```python
from build123d import *

# Parameters (mm, degrees)
SKETCH1_R           = 37.5
SKETCH1_R_2         = 21.5
BOSS_EXTRUDE1_DEPTH = 4
SKETCH2_R           = 29.5
SKETCH2_R_2         = 21.5
BOSS_EXTRUDE2_DEPTH = 79.3
SKETCH3_R           = 1.55
CUT_EXTRUDE1_DEPTH  = 96.399109011
CIRPATTERN1_COUNT   = 3
SKETCH4_R           = 2
CUT_EXTRUDE2_DEPTH  = 6
CIRPATTERN2_COUNT   = 4


with BuildPart() as part:
    # Sketch1 → Boss-Extrude1 (new body)
    with BuildSketch(Plane(origin=(0, 0, 0), x_dir=(1, 0, 0), z_dir=(0, 1, 0))):
        with Locations(Location((0, 0, 0), (0, 0, 270))):
            Circle(SKETCH1_R)
        with Locations(Location((0, 0, 0), (0, 0, 270))):
            Circle(SKETCH1_R_2, mode=Mode.SUBTRACT)
    extrude(amount=BOSS_EXTRUDE1_DEPTH)

    # Sketch2 → Boss-Extrude2 (add)
    with BuildSketch(Plane(origin=(0, 4, 0), x_dir=(1, 0, 0), z_dir=(0, 1, 0))):
        with Locations(Location((0, 0, 0), (0, 0, 270))):
            Circle(SKETCH2_R)
        with Locations(Location((0, 0, 0), (0, 0, 270))):
            Circle(SKETCH2_R_2, mode=Mode.SUBTRACT)
    extrude(amount=BOSS_EXTRUDE2_DEPTH)

    # Sketch3 → Cut-Extrude1 (cut, through all)
    with BuildSketch(Plane(origin=(0, 4, 0), x_dir=(1, 0, 0), z_dir=(0, 1, 0))):
        with Locations(Location((0, 33.5, 0), (0, 0, 270))):
            Circle(SKETCH3_R)
    cut_extrude1 = extrude(amount=-CUT_EXTRUDE1_DEPTH, mode=Mode.SUBTRACT)

    # CirPattern1: Cut-Extrude1 ×3 about axis
    cirpattern1_axis = Axis((0, 0, 0), (0, 1, 0))
    for i in range(1, CIRPATTERN1_COUNT):
        add(cut_extrude1.rotate(cirpattern1_axis, i * 360 / CIRPATTERN1_COUNT), mode=Mode.SUBTRACT)

    # Sketch4 → Cut-Extrude2 (cut)
    with BuildSketch(Plane(origin=(0, 83.3, 0), x_dir=(1, 0, 0), z_dir=(0, 1, 0))):
        with Locations(Location((-22.083647797, 12.75, 0), (0, 0, 270))):
            Circle(SKETCH4_R)
    cut_extrude2 = extrude(amount=-CUT_EXTRUDE2_DEPTH, mode=Mode.SUBTRACT)

    # CirPattern2: Cut-Extrude2 ×4 about axis
    cirpattern2_axis = Axis((0, 0, 0), (0, 1, 0))
    for i in range(1, CIRPATTERN2_COUNT):
        add(cut_extrude2.rotate(cirpattern2_axis, i * 360 / CIRPATTERN2_COUNT), mode=Mode.SUBTRACT)


solid = part.part
```
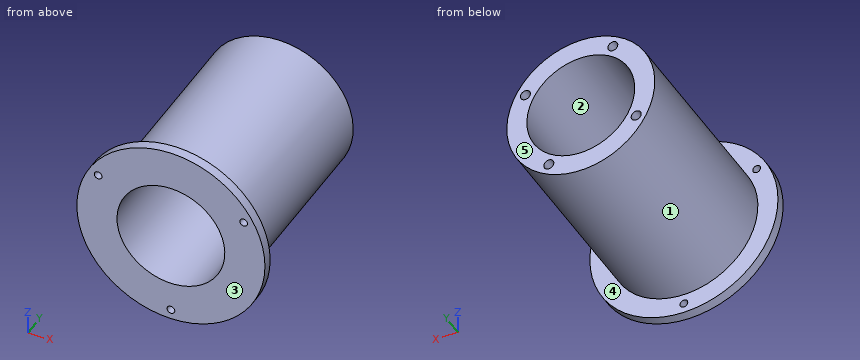
Could you check a few things on this model? Use its own coordinates, in mm. Face numbers are marked on the shaded views. A direction names the side the tool comes from. Round coordinates to 2 decimals unless told otherwise and drop trailing zeros. Write each loop counter-clockwise with the first axis right and the second up, starting at its lowest first coordinate (ties: lowest second). Pieces come first, ordered by that corner, then holes.
(1) Suppose I cut it at C-C on z = 12.75. Write out the boundary of the cut face in (x, y), and give its area (3 significant figures).
Findings below:
outline: (-35.27, 0) - (-17.31, 0) - (-17.31, 83.3) - (-26.6, 83.3) - (-26.6, 4) - (-35.27, 4) - close; (17.31, 0) - (35.27, 0) - (35.27, 4) - (26.6, 4) - (26.6, 83.3) - (24.08, 83.3) - (24.08, 77.3) - (20.08, 77.3) - (20.08, 83.3) - (17.31, 83.3) - close
area: 1,590 mm2
(2) Suppose I cut it at A-A on x = 0. Write out the boundary of the cut face in (y, z).
Findings below:
outline: (0, -37.5) - (4, -37.5) - (4, -35.05) - (0, -35.05) - close; (0, -31.95) - (4, -31.95) - (4, -29.5) - (83.3, -29.5) - (83.3, -21.5) - (0, -21.5) - close; (0, 21.5) - (83.3, 21.5) - (83.3, 29.5) - (4, 29.5) - (4, 37.5) - (0, 37.5) - close
(3) Which directions (+Z, -Z, +X, -X, +Y, -Y) give clear straight access to the entire face, cutting with the end or side of a thin tool? Please do the marked faces 4 and 5.
Findings below:
face 4: +Y
face 5: +Z, -Z, +X, -X, +Y
(4) If I drill on probe 1 along X at (y, z) = (1.35, 16.75); probe 2 along Y at (x, z) = (-30, 20.5); probe 3 along Z at (x, y) = (8, 32.5), over which ranges is the centre line in solid material (lowest first)?
Findings below:
probe 1: x = -33.55 to -30.56, -27.46 to -13.48, 13.48 to 27.46, 30.56 to 33.55
probe 2: y = 0 to 4
probe 3: z = -28.39 to -19.96, 19.96 to 28.39
(5) Suppose I cut it at B-B on x = 8.5. Write out the boundary of the cut face in (y, z).
Findings below:
outline: (0, -36.52) - (4, -36.52) - (4, -28.25) - (83.3, -28.25) - (83.3, -19.75) - (0, -19.75) - close; (0, 19.75) - (83.3, 19.75) - (83.3, 28.25) - (4, 28.25) - (4, 36.52) - (0, 36.52) - close
(6) Suppose I cut it at D-D on y = 58.5. Write out the boundary of the cut face in (x, z), and give its area (3 significant figures).
Findings below:
outline: circle Ø59 at (0, 0); hole circle Ø43 at (0, 0)
area: 1,280 mm2
(7) Thinking about a two-plate mould opening in Z: for the marked faces 1, 2 and 3, which applies, +Z half, -Z half, draft (parallel to the pull), parting line (faces both ways), or undercut?
Findings below:
face 1: parting line
face 2: undercut
face 3: draft
(8) For pin 1 (3 mm diameter, centred on x = 13, z = -22, fed in from +Y); pin 2 (8 mm diameter, centred on y = 19.5, z = -24, fed in from -X); pin 3 (10 mm diameter, centred on y = 74, z = -17.5, fed in from +X), each with a flat end and sliding along its axis, tell me the tip position at first contact or that it passes through.
Findings below:
pin 1: stops at y = 77.3
pin 2: stops at x = -21.69
pin 3: stops at x = 26.72
